from build123d import *

# Parameters (mm, degrees)
SKETCH1_R           = 1.3
BOSS_EXTRUDE1_DEPTH = 2
SKETCH2_W           = 15
SKETCH2_H           = 22
CUT_EXTRUDE1_DEPTH  = 2
FILLET1_R           = 1
SKETCH3_R           = 1.3
CUT_EXTRUDE2_DEPTH  = 2
SKETCH4_W           = 22
SKETCH4_H           = 6
CUT_EXTRUDE3_DEPTH  = 2
FILLET2_R           = 3


with BuildPart() as part:
    # Sketch1 → Boss-Extrude1 (new body)
    with BuildSketch(Plane(origin=(0, 0, 0), x_dir=(1, 0, 0), z_dir=(0, 1, 0))):
        Polygon((0, -80), (69.282032303, -40), (69.282032303, 40), (0, 80), (-69.282032303, 40), (-69.282032303, -40), align=None)
        with Locations(Location((65.282032303, 13.5, 0), (0, 0, 270))):
            Circle(SKETCH1_R, mode=Mode.SUBTRACT)
        with Locations(Location((57.282032303, 13.5, 0), (0, 0, 270))):
            Circle(SKETCH1_R, mode=Mode.SUBTRACT)
        with Locations(Location((51.782032303, 8, 0), (0, 0, 270))):
            Circle(SKETCH1_R, mode=Mode.SUBTRACT)
        with Locations(Location((51.782032303, -8, 0), (0, 0, 270))):
            Circle(SKETCH1_R, mode=Mode.SUBTRACT)
        with Locations(Location((57.282032303, -13.5, 0), (0, 0, 270))):
            Circle(SKETCH1_R, mode=Mode.SUBTRACT)
        with Locations(Location((65.282032303, -13.5, 0), (0, 0, 270))):
            Circle(SKETCH1_R, mode=Mode.SUBTRACT)
        with Locations(Location((32.819219382, -40.844555434, 0), (0, 0, 270))):
            Circle(SKETCH1_R, mode=Mode.SUBTRACT)
        with Locations(Location((20.9496732, -63.285898385, 0), (0, 0, 270))):
            Circle(SKETCH1_R, mode=Mode.SUBTRACT)
        with Locations(Location((16.9496732, -56.357695155, 0), (0, 0, 270))):
            Circle(SKETCH1_R, mode=Mode.SUBTRACT)
        with Locations(Location((18.962812921, -48.844555434, 0), (0, 0, 270))):
            Circle(SKETCH1_R, mode=Mode.SUBTRACT)
        with Locations(Location((44.332359102, -49.785898385, 0), (0, 0, 270))):
            Circle(SKETCH1_R, mode=Mode.SUBTRACT)
        with Locations(Location((40.332359102, -42.857695155, 0), (0, 0, 270))):
            Circle(SKETCH1_R, mode=Mode.SUBTRACT)
        with Locations(Location((-44.332359102, -49.785898385, 0), (0, 0, 270))):
            Circle(SKETCH1_R, mode=Mode.SUBTRACT)
        with Locations(Location((-40.332359102, -42.857695155, 0), (0, 0, 270))):
            Circle(SKETCH1_R, mode=Mode.SUBTRACT)
        with Locations(Location((-32.819219382, -40.844555434, 0), (0, 0, 270))):
            Circle(SKETCH1_R, mode=Mode.SUBTRACT)
        with Locations(Location((-18.962812921, -48.844555434, 0), (0, 0, 270))):
            Circle(SKETCH1_R, mode=Mode.SUBTRACT)
        with Locations(Location((-16.9496732, -56.357695155, 0), (0, 0, 270))):
            Circle(SKETCH1_R, mode=Mode.SUBTRACT)
        with Locations(Location((-20.9496732, -63.285898385, 0), (0, 0, 270))):
            Circle(SKETCH1_R, mode=Mode.SUBTRACT)
        with Locations(Location((18.962812921, 48.844555434, 0), (0, 0, 270))):
            Circle(SKETCH1_R, mode=Mode.SUBTRACT)
        with Locations(Location((44.332359102, 49.785898385, 0), (0, 0, 270))):
            Circle(SKETCH1_R, mode=Mode.SUBTRACT)
        with Locations(Location((40.332359102, 42.857695155, 0), (0, 0, 270))):
            Circle(SKETCH1_R, mode=Mode.SUBTRACT)
        with Locations(Location((32.819219382, 40.844555434, 0), (0, 0, 270))):
            Circle(SKETCH1_R, mode=Mode.SUBTRACT)
        with Locations(Location((20.9496732, 63.285898385, 0), (0, 0, 270))):
            Circle(SKETCH1_R, mode=Mode.SUBTRACT)
        with Locations(Location((16.9496732, 56.357695155, 0), (0, 0, 270))):
            Circle(SKETCH1_R, mode=Mode.SUBTRACT)
        with Locations(Location((-65.282032303, 13.5, 0), (0, 0, 270))):
            Circle(SKETCH1_R, mode=Mode.SUBTRACT)
        with Locations(Location((-20.9496732, 63.285898385, 0), (0, 0, 270))):
            Circle(SKETCH1_R, mode=Mode.SUBTRACT)
        with Locations(Location((-16.9496732, 56.357695155, 0), (0, 0, 270))):
            Circle(SKETCH1_R, mode=Mode.SUBTRACT)
        with Locations(Location((-18.962812921, 48.844555434, 0), (0, 0, 270))):
            Circle(SKETCH1_R, mode=Mode.SUBTRACT)
        with Locations(Location((-32.819219382, 40.844555434, 0), (0, 0, 270))):
            Circle(SKETCH1_R, mode=Mode.SUBTRACT)
        with Locations(Location((-44.332359102, 49.785898385, 0), (0, 0, 270))):
            Circle(SKETCH1_R, mode=Mode.SUBTRACT)
        with Locations(Location((-40.332359102, 42.857695155, 0), (0, 0, 270))):
            Circle(SKETCH1_R, mode=Mode.SUBTRACT)
        with Locations(Location((-57.282032303, 13.5, 0), (0, 0, 270))):
            Circle(SKETCH1_R, mode=Mode.SUBTRACT)
        with Locations(Location((-51.782032303, 8, 0), (0, 0, 270))):
            Circle(SKETCH1_R, mode=Mode.SUBTRACT)
        with Locations(Location((-51.782032303, -8, 0), (0, 0, 270))):
            Circle(SKETCH1_R, mode=Mode.SUBTRACT)
        with Locations(Location((-57.282032303, -13.5, 0), (0, 0, 270))):
            Circle(SKETCH1_R, mode=Mode.SUBTRACT)
        with Locations(Location((-65.282032303, -13.5, 0), (0, 0, 270))):
            Circle(SKETCH1_R, mode=Mode.SUBTRACT)
    extrude(amount=BOSS_EXTRUDE1_DEPTH)

    # Sketch2 → Cut-Extrude1 (cut)
    with BuildSketch(Plane(origin=(0, 2, 0), x_dir=(1, 0, 0), z_dir=(0, 1, 0))):
        with Locations((61.782032303, 0)):
            Rectangle(SKETCH2_W, SKETCH2_H)
        Polygon((44.167295593, -54.5), (36.667295593, -41.509618943), (17.61473671, -52.509618943), (25.11473671, -65.5), align=None)
        Polygon((-25.11473671, -65.5), (-44.167295593, -54.5), (-36.667295593, -41.509618943), (-17.61473671, -52.509618943), align=None)
        Polygon((25.11473671, 65.5), (17.61473671, 52.509618943), (36.667295593, 41.509618943), (44.167295593, 54.5), align=None)
        Polygon((-44.167295593, 54.5), (-25.11473671, 65.5), (-17.61473671, 52.509618943), (-36.667295593, 41.509618943), align=None)
        with Locations((-61.782032303, 0)):
            Rectangle(SKETCH2_W, SKETCH2_H)
    extrude(amount=-CUT_EXTRUDE1_DEPTH, mode=Mode.SUBTRACT)

    # Fillet1
    fillet1_edges = [part.edges().sort_by_distance(p)[0] for p in [
        (69.282032303, 1, -11),
        (69.282032303, 1, 11),
        (44.167295593, 1, 54.5),
        (25.11473671, 1, 65.5),
        (-25.11473671, 1, 65.5),
        (-44.167295593, 1, 54.5),
        (25.11473671, 1, -65.5),
        (44.167295593, 1, -54.5),
        (-44.167295593, 1, -54.5),
        (-25.11473671, 1, -65.5),
        (-69.282032303, 1, 11),
        (-69.282032303, 1, -11),
        (-69.282032303, 1, -40),
        (0, 1, -80),
        (69.282032303, 1, -40),
        (69.282032303, 1, 40),
        (0, 1, 80),
        (-69.282032303, 1, 40),
    ]]
    fillet(fillet1_edges, radius=FILLET1_R)

    # Sketch3 → Cut-Extrude2 (cut)
    with BuildSketch(Plane(origin=(0, 2, 0), x_dir=(1, 0, 0), z_dir=(0, 1, 0))):
        with Locations(Location((-22.836753878, -38.995299462, 0), (0, 0, 270))):
            Circle(SKETCH3_R)
        with Locations(Location((-22.836753878, 19.004700538, 0), (0, 0, 270))):
            Circle(SKETCH3_R)
        with Locations(Location((26.163246122, 19.004700538, 0), (0, 0, 270))):
            Circle(SKETCH3_R)
        with Locations(Location((26.163246122, -38.995299462, 0), (0, 0, 270))):
            Circle(SKETCH3_R)
    extrude(amount=-CUT_EXTRUDE2_DEPTH, mode=Mode.SUBTRACT)

    # Sketch4 → Cut-Extrude3 (cut)
    with BuildSketch(Plane(origin=(0, 2, 0), x_dir=(1, 0, 0), z_dir=(0, 1, 0))):
        with Locations((0, 64)):
            Rectangle(SKETCH4_W, SKETCH4_H)
    extrude(amount=-CUT_EXTRUDE3_DEPTH, mode=Mode.SUBTRACT)

    # Fillet2
    fillet2_edges = [part.edges().sort_by_distance(p)[0] for p in [
        (11, 1, -67),
        (-11, 1, -67),
        (-11, 1, -61),
        (11, 1, -61),
    ]]
    fillet(fillet2_edges, radius=FILLET2_R - 0.0001)  # a hair under: the kernel refuses the full size


solid = part.part
The listing builds one solid part. Answer for the finished solid, in the listing's coordinates (mm). A direction names the side the tool comes from. Give positions to 0.01 mm unless a question says otherwise; leave off trailing zeros. Loops run counter-clockwise (first coordinate to the right, second up) from the corner with the lowest first, then second, coordinate; pieces in that order, holes last. Notation, with made-up numbers: (65, 8) - (70, 8) arc R9 cw to (70, 13) - close; hole circle Ø1 at (-14.75, -33). An arc over 180 degrees is marked (long way). Answer as a JSON object with one key per item and string values.
1. Find the intervals of material crossed by L1, parallel to X at y = 1.5, z = 8; L2, parallel to X at y = 0.5, z = 13.5; L3, parallel to X at y = 1.95, z = -56, in increasing order. Write a range as [from, to].
Determined:
{"L1": "[-54.28, -53.08], [-50.48, 50.48], [53.08, 54.28]", "L2": "[-69.28, -66.58], [-63.98, -58.58], [-55.98, 55.98], [58.58, 63.98], [66.58, 69.28]", "L3": "[-19.63, -18.2], [-15.7, 15.7], [18.2, 19.63]"}
2. A cutting plane is placed at C-C (y = 1.05). Give the number of separate pieces and of enclosed holes in the cut face, then the cut area to 3 significant figures.
Determined:
{"separate pieces": "1", "enclosed holes": "41", "area": "14,300 mm²"}
3. A cutting plane is placed at B-B (z = 2). Write down the section's boundary in (x, y), then the cut area to 3 significant figures.
Determined:
{"outline": "(-54.28, 0) - (54.28, 0) - (54.28, 2) - (-54.28, 2) - close", "area": "217 mm²"}
4. For a pull along Z with two mould halves and no side action, classify faces 1 (the flat face through (-1, 0, -1)), 2 (the flat face through (-40.12, 1.01, -47.49)), 3 (the flat face through (56.74, 0.99, 47.24)), 4 (the flat face through (-21.164, 1.014, -58.657)) as pulls with the +Z half, pulls with the -Z half, needs draft (parallel to the pull), parting line crosses it, or undercut.
Determined:
{"face 1": "needs draft", "face 2": "pulls with the -Z half", "face 3": "pulls with the +Z half", "face 4": "undercut"}
5. A cutting plane is placed at A-A (x = 2.5). Write down the section's boundary in (y, z), then the cut area to 3 significant figures.
Determined:
{"outline": "(0, -78.56) - (2, -78.56) - (2, -67) - (0, -67) - close; (0, -61) - (2, -61) - (2, 78.56) - (0, 78.56) - close", "area": "302 mm²"}
6. For faces 5 (the flat face through (40.12, 1.01, -47.49)), 6 (the flat face through (-1, 2, -1)), 7 (the flat face through (-27.008, 1.014, -47.087)), 8 (the flat face through (-40.22, 1.01, 47.66)), 9 (the flat face through (12.54, 0.99, -72.76)), determine the directions among +Z, -Z, +X, -X, +Y, -Y from which every point of the face is accessible in a straight line to the end or side of a thin tool.
Determined:
{"face 5": "-Z, +Y, -Y", "face 6": "+Z, -Z, +X, -X, +Y", "face 7": "+Y, -Y", "face 8": "+Z, +Y, -Y", "face 9": "-Z, +X, +Y, -Y"}
7. A flat-ended cylindrical pin translates along its axis: pin 1 Ø0.6 at (y, z) = (1, -3) entering from -X. Find the tip coordinate at first contact, or state that the pin passes through.
Determined:
{"pin 1": "x = -54.28"}
